Design review of the part shown in the three views and the two pictorial views. Dimensions are in mm from the part's minimum x, y and z. Coordinates: 2 decimals unless noted, no trailing zeros. Order: outer loops, then holes, each group sorted by start corner. A loop starts at its lowest first (then second) coordinate and runs counter-clockwise, first axis right, second up. Notation, with made-up numbers: (19.5, 66.5) -> (74.5, 66.5) arc R7 cw to (74.5, 76.5) -> close; hole circle Ø9 at (38.5, 45.5). An arc over 180 degrees is marked (long way). Answer as a JSON object with one key per item and string values. Group by question number.
1) For pin 1 (7 mm diameter, centred on x = 175, z = 335, fed in from +Y); pin 2 (12 mm diameter, centred on y = 15, z = 251.5, fed in from -X); pin 3 (1 mm diameter, centred on y = 11, z = 127.5, fed in from +X); pin 4 (1 mm diameter, centred on y = 24.5, z = 142.5, fed in from +X), all flat-tipped, find the tip position at first contact; note any pin that passes through.
2) Add section A-A, the plane z = 217. Write out the cut boundary in (x, y).
3) Draft analysis for pull direction Z (two halves, no side actions). For the marked faces 1, 2 and 3, state which applies: +Z half, -Z half, draft (parallel to the pull), parting line (faces both ways), or undercut.
4) Wall thickness on L1, parallel to X at y = 12.5, z = 175; L2, parallel to X at y = 2.25, z = 195; L3, parallel to Z at x = 206.5, y = 22: over which ranges is each line inside the solid? List them lowest first.
5) Add section C-C, the plane y = 11.5. Write out the cut boundary in (x, z), then the cut area to 3 significant figures.
6) Add section B-B, the plane x = 187.5. Write out the cut boundary in (y, z), then the cut area to 3 significant figures.
7) Add section D-D, the plane z = 318. Write out the cut boundary in (x, y).
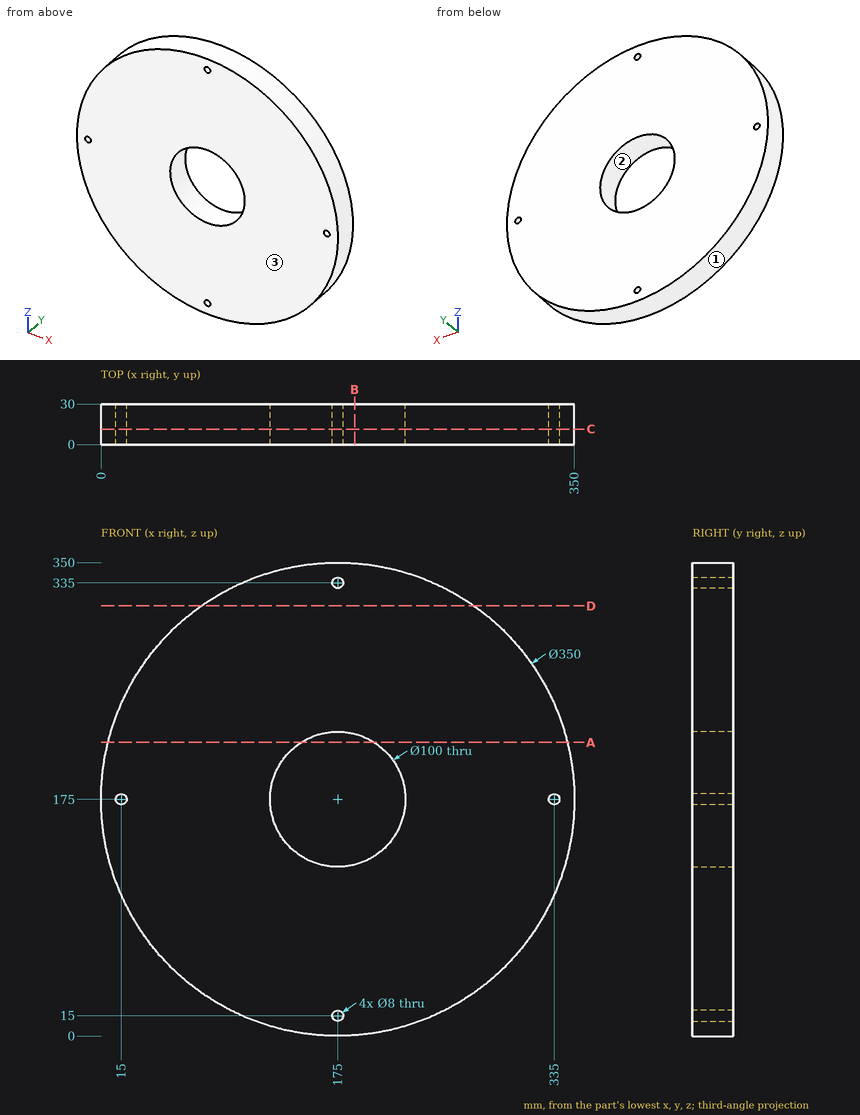
Output values:
{
 "1": {"pin 1": "passes through", "pin 2": "stops at x = 14.83", "pin 3": "stops at x = 343.57", "pin 4": "stops at x = 347.05"},
 "2": {"outline": "(5.11, 0) -> (147.87, 0) -> (147.87, 30) -> (5.11, 30) -> close; (202.13, 0) -> (344.89, 0) -> (344.89, 30) -> (202.13, 30) -> close"},
 "3": {"face 1": "parting line", "face 2": "undercut", "face 3": "draft"},
 "4": {"L1": "x = 0 to 11, 19 to 125, 225 to 331, 339 to 350", "L2": "x = 1.15 to 129.17, 220.83 to 348.85", "L3": "z = 2.86 to 136.17, 213.83 to 347.14"},
 "5": {"outline": "circle Ø350 at (175, 175); hole circle Ø8 at (15, 175); hole circle Ø100 at (175, 175); hole circle Ø8 at (175, 15); hole circle Ø8 at (175, 335); hole circle Ø8 at (335, 175)", "area": "88,200 mm²"},
 "6": {"outline": "(0, 0.45) -> (30, 0.45) -> (30, 126.59) -> (0, 126.59) -> close; (0, 223.41) -> (30, 223.41) -> (30, 349.55) -> (0, 349.55) -> close", "area": "7,570 mm²"},
 "7": {"outline": "(74.12, 0) -> (275.88, 0) -> (275.88, 30) -> (74.12, 30) -> close"}
}
